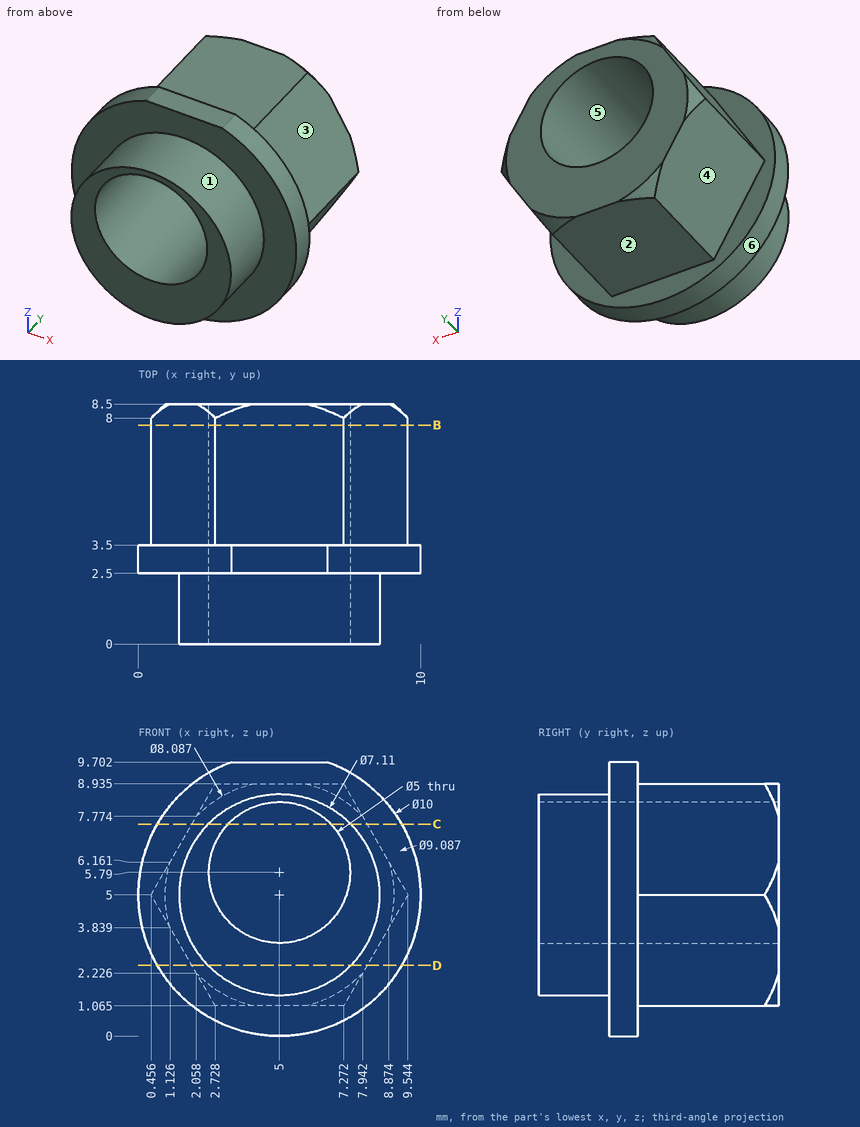
Study the drawing (mm; zero at the part's minimum x, y, z) and answer. A direction names the side the tool comes from. Round coordinates to 2 decimals unless told otherwise and drop trailing zeros. Loops run counter-clockwise (first coordinate to the right, second up) from the corner with the lowest first, then second, coordinate; pieces in that order, holes last. Notation, with made-up numbers: M 10,-1 L 55,-1 A8 ccw 55,13 Z; hole C 84.5,16.5 d10. An arc over 180 degrees is marked long. One line per question, with ' | ' between items.
Q1. The mould has two halves that part along Z. Classify the marked faces 4, 5 and 6: +Z half, -Z half, draft (parallel to the pull), parting line (faces both ways), or undercut.
Conclusion:
face 4: -Z half | face 5: undercut | face 6: parting line
Q2. Consider line 1 along Z through (x, y) = (5, 5) (1 decimal); line 2 along X through (y, z) = (7.25, 5.5) (1 decimal); line 3 along Y through (x, z) = (7, 8). Determine where each line is inside the solid, lowest interval first. Write a range as from..to.
Conclusion:
line 1: z = 1.1..3.3, 8.3..8.9 | line 2: x = 0.7..2.5, 7.5..9.3 | line 3: y = 2.5..8.5
Q3. Find section B-B, the plane y = 7.75. Give the vertices of the cut face in (x, z) (1 decimal), then the cut area to 3 significant figures.
Conclusion:
outline: M 0.5,5 L 2.7,1.1 L 7.3,1.1 L 9.5,5 L 7.3,8.9 L 2.7,8.9 Z; hole C 5,5.8 d5 | area: 34.0 mm2
Q4. Find section C-C, the plane z = 7.5. Give the vertices of the cut face in (x, y).
Conclusion:
outline: M 0.67,2.5 L 2.47,2.5 L 2.47,0 L 3.18,0 L 3.18,8.5 L 1.9,8.5 L 1.9,3.5 L 0.67,3.5 Z; M 6.82,0 L 7.53,0 L 7.53,2.5 L 9.33,2.5 L 9.33,3.5 L 8.1,3.5 L 8.1,8.5 L 6.82,8.5 Z
Q5. A tool of negligible diameter and unlimited length cuts with its end or side. For the marked faces 1, 2 and 3, from which of +Z, -Z, +X, -X, +Y, -Y can it reach the whole face along a straight path? Write none if from no direction.
Conclusion:
face 1: -Y | face 2: -Z, +X, -X, +Y | face 3: +Z, +X, +Y
Q6. Find section D-D, the plane z = 2.5. Give the vertices of the cut face in (x, y), then the cut area to 3 significant figures.
Conclusion:
outline: M 0.67,2.5 L 2.47,2.5 L 2.47,0 L 7.53,0 L 7.53,2.5 L 9.33,2.5 L 9.33,3.5 L 8.1,3.5 L 8.1,8.5 L 1.9,8.5 L 1.9,3.5 L 0.67,3.5 Z | area: 52.3 mm2
Q7. Each of these flat-tipped pins is pushed along its axis until it touches: pin 1 Ø3 at (x, z) = (4.5, 6) entering from -Y; pin 2 Ø3.5 at (x, y) = (6, 6.5) entering from -Z (1 decimal); pin 3 Ø5 at (x, y) = (6, 7) entering from +Z (1 decimal); pin 4 Ø5 at (x, y) = (8.5, 4) entering from -Z. Where does it stop, or does it pass through?
Conclusion:
pin 1: passes through | pin 2: stops at z = 1.1 | pin 3: stops at z = 8.9 | pin 4: stops at z = 0.11
